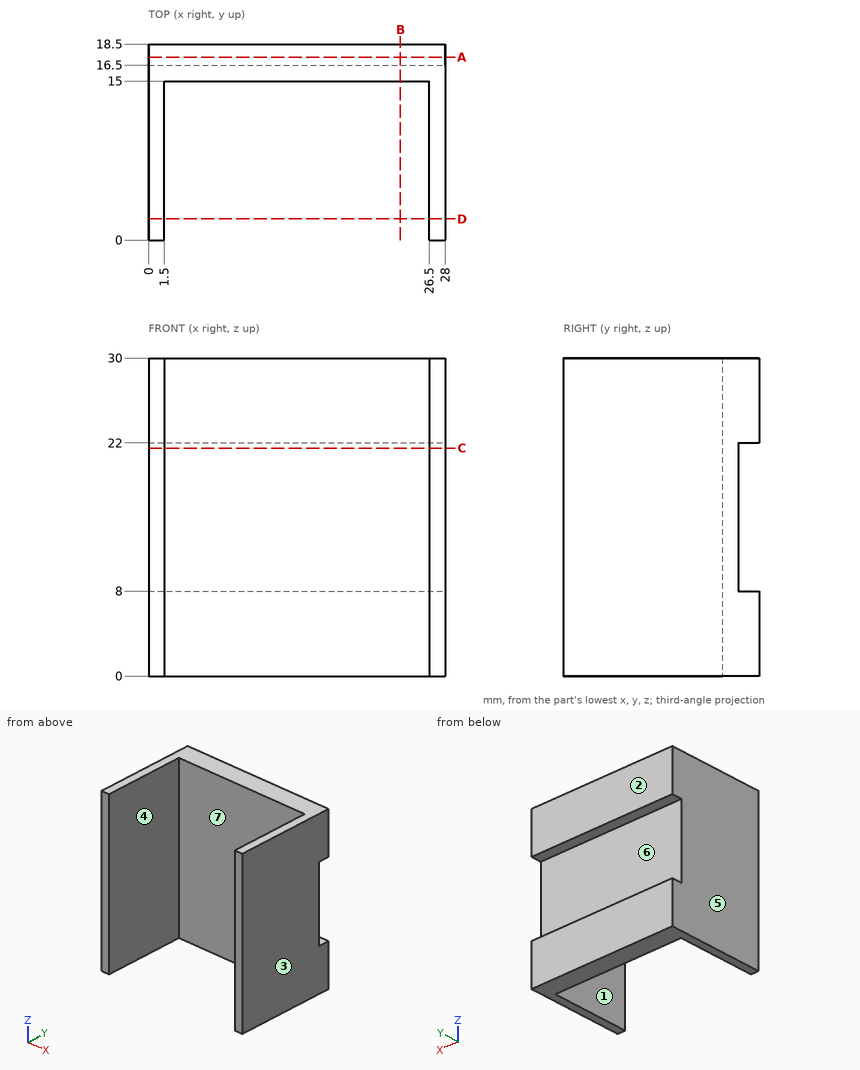
Geometry: see drawing. Coordinates: mm, zero at the bounding-box minimum. A direction names the side the tool comes from. Round coordinates to 2 decimals unless told otherwise and drop trailing zeros. Loops run counter-clockwise (first coordinate to the right, second up) from the corner with the lowest first, then second, coordinate; pieces in that order, holes last.
(1) Material intervals for probe 1 along X at (y, z) = (7.75, 4.75); probe 2 along Y at (x, z) = (20, 15.25); probe 3 along Y at (x, z) = (23.75, 6), sorted ascending.
From the geometry:
probe 1: x = 0 to 1.5, 26.5 to 28
probe 2: y = 15 to 16.5
probe 3: y = 15 to 18.5
(2) Section query D-D (y = 2). Output: boundary loops of the cut face in (x, z), and give its area (3 significant figures).
From the geometry:
outline: (0, 0) - (1.5, 0) - (1.5, 30) - (0, 30) - close; (26.5, 0) - (28, 0) - (28, 30) - (26.5, 30) - close
area: 90.0 mm2
(3) Section query C-C (z = 21.5). Output: boundary loops of the cut face in (x, y).
From the geometry:
outline: (0, 0) - (1.5, 0) - (1.5, 15) - (26.5, 15) - (26.5, 0) - (28, 0) - (28, 16.5) - (0, 16.5) - close
(4) Access query for the marked faces 5, 6 and 7. Directions: +Z, -Z, +X, -X, +Y, -Y. A direction counts if a zero-diameter tool reaches every point of the face in a straight line with its end or side. Return the directions, or none.
From the geometry:
face 5: +Z, -Z, -X, +Y, -Y
face 6: +X, -X, +Y
face 7: +Z, -Z, -Y
(5) Pull-direction query (X, two-part tool) for the marked faces 1, 2, 3 and 4; classes: +X half, -X half, draft (parallel to the pull), parting line (faces both ways), or undercut.
From the geometry:
face 1: undercut
face 2: draft
face 3: +X half
face 4: undercut
(6) Contact query for flat-ended pins moving along their axis: pin 1 Ø10 at (x, z) = (4, 18) entering from -Y; pin 2 Ø7 at (x, z) = (18.5, 13) entering from +Y; pin 3 Ø2 at (x, z) = (15.5, 19) entering from -Y. Output: stop coordinate, or through.
From the geometry:
pin 1: stops at y = 0
pin 2: stops at y = 16.5
pin 3: stops at y = 15
(7) Section query B-B (x = 23.75). Output: boundary loops of the cut face in (y, z).
From the geometry:
outline: (15, 0) - (18.5, 0) - (18.5, 8) - (16.5, 8) - (16.5, 22) - (18.5, 22) - (18.5, 30) - (15, 30) - close
(8) Section query A-A (y = 17.25). Output: boundary loops of the cut face in (x, z).
From the geometry:
outline: (0, 0) - (28, 0) - (28, 8) - (0, 8) - close; (0, 22) - (28, 22) - (28, 30) - (0, 30) - close
